For this review, take the finished solid that the model builds, in its own axes (mm). Face numbers are marked on the shaded views. A direction names the side the tool comes from. Round coordinates to 2 decimals unless told otherwise and drop trailing zeros. Order: outer loops, then holes, each group sorted by start corner. A loop starts at its lowest first (then second) coordinate and runs counter-clockwise, first axis right, second up. Notation, with made-up numbers: (77.25, 14.5) -> (117.25, 14.5) arc R7 cw to (117.25, 27.5) -> close; hole circle Ø9 at (-35.75, -22.75). An arc over 180 degrees is marked (long way). Answer in a Markdown table with one row per item.
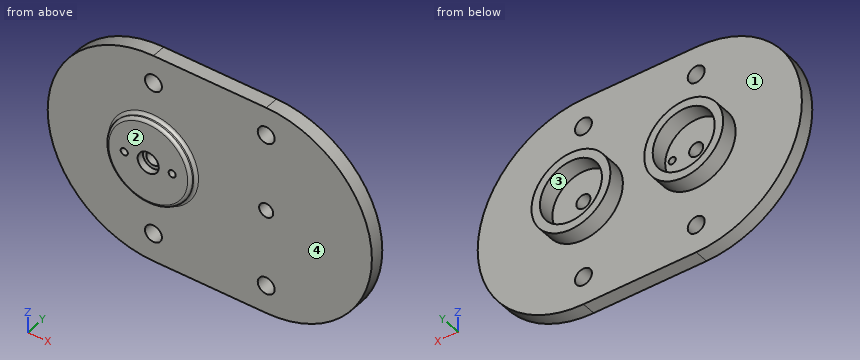
```python
from build123d import *

# Parameters (mm, degrees)
SALIENTE_EXTRUIR1_DEPTH = 2.5
CROQUIS2_R              = 14
CROQUIS2_R_2            = 11
SALIENTE_EXTRUIR2_DEPTH = 6
CROQUIS8_R              = 15
CROQUIS8_R_2            = 3.75
SALIENTE_EXTRUIR4_DEPTH = 2.5
REDONDEO2_R             = 1
CORTAR_EXTRUIR1_REACH   = 71.056
CROQUIS6_R              = 1.265
CROQUIS6_R_2            = 2.5
CROQUIS6_R_3            = 3


with BuildPart() as part:
    # Croquis1 → Saliente-Extruir1 (new, symmetric)
    with BuildSketch(Plane(origin=(0, 0, 0), x_dir=(1, 0, 0), z_dir=(0, 1, 0))):
        with BuildLine():
            Line((-20, 37.5), (20, 37.5))
            ThreePointArc((20, 37.5), (57.5, 0), (20, -37.5))
            Line((20, -37.5), (-20, -37.5))
            ThreePointArc((-20, -37.5), (-57.5, 0), (-20, 37.5))
        make_face()
    extrude(amount=SALIENTE_EXTRUIR1_DEPTH, both=True)

    # Croquis2 → Saliente-Extruir2 (add)
    # profile 1 of 2: a face of its own
    with BuildSketch(Plane(origin=(0, 2.5, 0), x_dir=(1, 0, 0), z_dir=(0, 1, 0))):
        with Locations(Location((-20, 0, 0), (0, 0, 270))):
            Circle(CROQUIS2_R)
        with Locations(Location((-20, 0, 0), (0, 0, 270))):
            Circle(CROQUIS2_R_2, mode=Mode.SUBTRACT)
    # profile 2 of 2: a face of its own
    with BuildSketch(Plane(origin=(0, 2.5, 0), x_dir=(1, 0, 0), z_dir=(0, 1, 0))):
        with Locations(Location((20, 0, 0), (0, 0, 270))):
            Circle(CROQUIS2_R)
        with Locations(Location((20, 0, 0), (0, 0, 270))):
            Circle(CROQUIS2_R_2, mode=Mode.SUBTRACT)
    extrude(amount=SALIENTE_EXTRUIR2_DEPTH)

    # Croquis8 → Saliente-Extruir4 (add)
    with BuildSketch(Plane.XZ.offset(2.5)):
        with Locations(Location((-20, 0, 0), (0, 0, 270))):
            Circle(CROQUIS8_R)
        with Locations(Location((-20, 0, 0), (0, 0, 270))):
            Circle(CROQUIS8_R_2, mode=Mode.SUBTRACT)
    extrude(amount=SALIENTE_EXTRUIR4_DEPTH)

    # Redondeo2
    redondeo2_edges = [part.edges().sort_by_distance(p)[0] for p in [
        (-20, -2.5, 15),
        (-20, -5, 15),
    ]]
    fillet(redondeo2_edges, radius=REDONDEO2_R)

    # Croquis6 → Cortar-Extruir1 (cut, up to next)
    with BuildSketch(Plane(origin=(0, 2.5, 0), x_dir=(1, 0, 0), z_dir=(0, 1, 0)), mode=Mode.PRIVATE) as cortar_extruir1_sk1:
        with Locations(Location((-28.5, 0, 0), (0, 0, 270))):
            Circle(CROQUIS6_R)
    cortar_extruir1_tool1 = extrude(cortar_extruir1_sk1.sketch, amount=-CORTAR_EXTRUIR1_REACH, mode=Mode.PRIVATE) & part.part
    # Croquis6 → Cortar-Extruir1 (cut, up to next)
    with BuildSketch(Plane(origin=(0, 2.5, 0), x_dir=(1, 0, 0), z_dir=(0, 1, 0)), mode=Mode.PRIVATE) as cortar_extruir1_sk2:
        with Locations(Location((-11.5, 0, 0), (0, 0, 270))):
            Circle(CROQUIS6_R)
    cortar_extruir1_tool2 = extrude(cortar_extruir1_sk2.sketch, amount=-CORTAR_EXTRUIR1_REACH, mode=Mode.PRIVATE) & part.part
    # Croquis6 → Cortar-Extruir1 (cut, up to next)
    with BuildSketch(Plane(origin=(0, 2.5, 0), x_dir=(1, 0, 0), z_dir=(0, 1, 0)), mode=Mode.PRIVATE) as cortar_extruir1_sk3:
        with Locations(Location((-20, 0, 0), (0, 0, 270))):
            Circle(CROQUIS6_R_2)
    cortar_extruir1_tool3 = extrude(cortar_extruir1_sk3.sketch, amount=-CORTAR_EXTRUIR1_REACH, mode=Mode.PRIVATE) & part.part
    # Croquis6 → Cortar-Extruir1 (cut, up to next)
    with BuildSketch(Plane(origin=(0, 2.5, 0), x_dir=(1, 0, 0), z_dir=(0, 1, 0)), mode=Mode.PRIVATE) as cortar_extruir1_sk4:
        with Locations(Location((20, 0, 0), (0, 0, 270))):
            Circle(CROQUIS6_R_2)
    cortar_extruir1_tool4 = extrude(cortar_extruir1_sk4.sketch, amount=-CORTAR_EXTRUIR1_REACH, mode=Mode.PRIVATE) & part.part
    # Croquis6 → Cortar-Extruir1 (cut, up to next)
    with BuildSketch(Plane(origin=(0, 2.5, 0), x_dir=(1, 0, 0), z_dir=(0, 1, 0)), mode=Mode.PRIVATE) as cortar_extruir1_sk5:
        with Locations(Location((-20, 27.5, 0), (0, 0, 270))):
            Circle(CROQUIS6_R_3)
    cortar_extruir1_tool5 = extrude(cortar_extruir1_sk5.sketch, amount=-CORTAR_EXTRUIR1_REACH, mode=Mode.PRIVATE) & part.part
    # Croquis6 → Cortar-Extruir1 (cut, up to next)
    with BuildSketch(Plane(origin=(0, 2.5, 0), x_dir=(1, 0, 0), z_dir=(0, 1, 0)), mode=Mode.PRIVATE) as cortar_extruir1_sk6:
        with Locations(Location((20, 27.5, 0), (0, 0, 270))):
            Circle(CROQUIS6_R_3)
    cortar_extruir1_tool6 = extrude(cortar_extruir1_sk6.sketch, amount=-CORTAR_EXTRUIR1_REACH, mode=Mode.PRIVATE) & part.part
    # Croquis6 → Cortar-Extruir1 (cut, up to next)
    with BuildSketch(Plane(origin=(0, 2.5, 0), x_dir=(1, 0, 0), z_dir=(0, 1, 0)), mode=Mode.PRIVATE) as cortar_extruir1_sk7:
        with Locations(Location((20, -27.5, 0), (0, 0, 270))):
            Circle(CROQUIS6_R_3)
    cortar_extruir1_tool7 = extrude(cortar_extruir1_sk7.sketch, amount=-CORTAR_EXTRUIR1_REACH, mode=Mode.PRIVATE) & part.part
    # Croquis6 → Cortar-Extruir1 (cut, up to next)
    with BuildSketch(Plane(origin=(0, 2.5, 0), x_dir=(1, 0, 0), z_dir=(0, 1, 0)), mode=Mode.PRIVATE) as cortar_extruir1_sk8:
        with Locations(Location((-20, -27.5, 0), (0, 0, 270))):
            Circle(CROQUIS6_R_3)
    cortar_extruir1_tool8 = extrude(cortar_extruir1_sk8.sketch, amount=-CORTAR_EXTRUIR1_REACH, mode=Mode.PRIVATE) & part.part
    add(cortar_extruir1_tool1.solids().sort_by_distance((-28.5, 2.5, 0))[0], mode=Mode.SUBTRACT)
    add(cortar_extruir1_tool2.solids().sort_by_distance((-11.5, 2.5, 0))[0], mode=Mode.SUBTRACT)
    add(cortar_extruir1_tool3.solids().sort_by_distance((-20, 2.5, 0))[0], mode=Mode.SUBTRACT)
    add(cortar_extruir1_tool4.solids().sort_by_distance((20, 2.5, 0))[0], mode=Mode.SUBTRACT)
    add(cortar_extruir1_tool5.solids().sort_by_distance((-20, 2.5, -27.5))[0], mode=Mode.SUBTRACT)
    add(cortar_extruir1_tool6.solids().sort_by_distance((20, 2.5, -27.5))[0], mode=Mode.SUBTRACT)
    add(cortar_extruir1_tool7.solids().sort_by_distance((20, 2.5, 27.5))[0], mode=Mode.SUBTRACT)
    add(cortar_extruir1_tool8.solids().sort_by_distance((-20, 2.5, 27.5))[0], mode=Mode.SUBTRACT)


solid = part.part
```
Q1. Take a section at C-C, the plane z = 27.5. Write out the cut boundary in (x, y).
Answer key:
| item | result |
|---|---|
| outline | (-45.5, -2.5) -> (-23, -2.5) -> (-23, 2.5) -> (-45.5, 2.5) -> close; (-17, -2.5) -> (17, -2.5) -> (17, 2.5) -> (-17, 2.5) -> close; (23, -2.5) -> (45.5, -2.5) -> (45.5, 2.5) -> (23, 2.5) -> close |
Q2. Take a section at D-D, the plane x = 7.5. Write out the cut boundary in (y, z).
Answer key:
| item | result |
|---|---|
| outline | (-2.5, -37.5) -> (2.5, -37.5) -> (2.5, -6.3) -> (8.5, -6.3) -> (8.5, 6.3) -> (2.5, 6.3) -> (2.5, 37.5) -> (-2.5, 37.5) -> close |
Q3. To check wall thickness, follow probe 1 along X at (y, z) = (-1.2, 0) (3 decimals); probe 2 along X at (y, z) = (-0.4, -27.5); probe 3 along Y at (x, z) = (48.5, 24). State the ranges of each line that lie inside material, in increasing order.
Answer key:
| item | result |
|---|---|
| probe 1 | x = -57.5 to -29.765, -27.235 to -22.5, -17.5 to -12.765, -10.235 to 17.5, 22.5 to 57.5 |
| probe 2 | x = -45.5 to -23, -17 to 17, 23 to 45.5 |
| probe 3 | y = -2.5 to 2.5 |
Q4. Take a section at A-A, the plane y = 1. Give the number of separate pieces and of enclosed holes in the cut face, then the cut area to 3 significant figures.
Answer key:
| item | result |
|---|---|
| separate pieces | 1 |
| enclosed holes | 8 |
| area | 7,260 mm^2 |
Q5. The part is to be moulded in two halves that separate along X. For the marked faces 3 and 4, say which applies: +X half, -X half, draft (parallel to the pull), parting line (faces both ways), or undercut.
Answer key:
| item | result |
|---|---|
| face 3 | undercut |
| face 4 | draft |
Q6. Tool access review of the marked faces 1 and 2: name each direction out of +Z, -Z, +X, -X, +Y, -Y from which nothing blocks a thin tool from reaching the whole face with its end or side.
Answer key:
| item | result |
|---|---|
| face 1 | +Y |
| face 2 | +Z, -Z, +X, -X, -Y |
Q7. Take a section at B-B, the plane y = 7.25. Write out the cut boundary in (x, z).
Answer key:
| item | result |
|---|---|
| outline | circle Ø28 at (-20, 0); circle Ø28 at (20, 0); hole circle Ø22 at (-20, 0); hole circle Ø22 at (20, 0) |
Q8. Clearance check with flat-ended pins moving along their axes: pin 1 Ø8 at (x, z) = (20, -27.5) entering from +Y; pin 2 Ø6 at (y, z) = (1, 21) entering from +X; pin 3 Ø6.5 at (x, z) = (20, 0) entering from -Y; pin 4 Ø3.5 at (x, z) = (20, 27.5) entering from -Y. State where each tip first meets the part, or that it passes through.
Answer key:
| item | result |
|---|---|
| pin 1 | stops at y = 2.5 |
| pin 2 | stops at x = 52.9 |
| pin 3 | stops at y = -2.5 |
| pin 4 | passes through |
